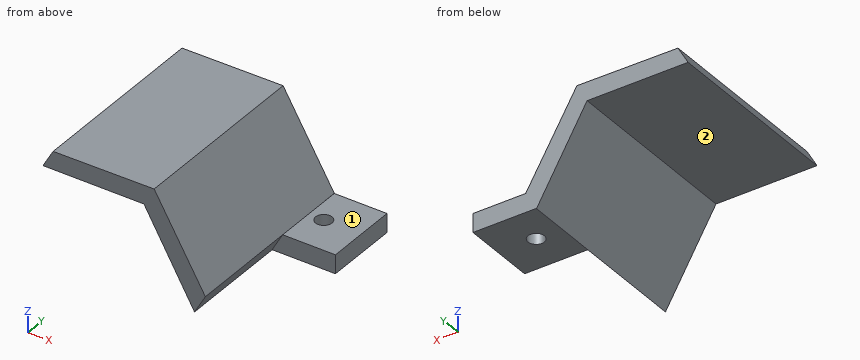
```python
from build123d import *

# Parameters (mm, degrees)
ESQUISSE3_W             = 20
ESQUISSE3_H             = 20
BOSS_EXTRU_2_DEPTH      = 5
ESQUISSE5_R             = 2.2
ENL_V_MAT_EXTRU_2_DEPTH = 5
BOSS_EXTRU_4_DEPTH      = 1
BOSS_EXTRU_4_DEPTH_BACK = 50
ENL_V_MAT_EXTRU_3_DEPTH = 52
ESQUISSE17_W            = 44.772761967
ESQUISSE17_H            = 32.67201549
ENL_V_MAT_EXTRU_4_DEPTH = 1


with BuildPart() as part:
    # Esquisse3 → Boss.-Extru.2 (new body)
    with BuildSketch(Plane.XY):
        with Locations((0.833384448, -1.552723646)):
            Rectangle(ESQUISSE3_W, ESQUISSE3_H)
    extrude(amount=BOSS_EXTRU_2_DEPTH)

    # Esquisse5 → Enlèv. mat.-Extru.2 (cut)
    with BuildSketch(Plane.XY.offset(5)):
        with Locations((0.833384448, -1.552723646)):
            Circle(ESQUISSE5_R)
    extrude(amount=-ENL_V_MAT_EXTRU_2_DEPTH, mode=Mode.SUBTRACT)

    # Esquisse15 → Boss.-Extru.4 (add, two sides: drawn at the far end of the back side and taken through both)
    with BuildSketch(Plane(origin=(0, 8.447276354, 0), x_dir=(1, 0, 0), z_dir=(0, 1, 0)).offset(-BOSS_EXTRU_4_DEPTH_BACK)):
        Polygon((-16.923746628, -28.293399859), (-3.242841841, -5.019846719), (-16.557877703, 18.464940943), (-43.553818352, 18.676175465), (-57.234723139, -4.597377675), (-43.919687277, -28.082165337), align=None)
    extrude(amount=BOSS_EXTRU_4_DEPTH + BOSS_EXTRU_4_DEPTH_BACK)

    # Esquisse16 → Enlèv. mat.-Extru.3 (cut)
    with BuildSketch(Plane(origin=(0, 9.447276354, 0), x_dir=(1, 0, 0), z_dir=(0, 1, 0))):
        Polygon((-3.971698256, 3.828685124), (-19.643043748, 30.972251739), (-50.985734731, 30.972251739), (-66.657080223, 3.828685124), (-50.985734731, -23.314881491), (-19.643043748, -23.314881491), align=None)
    extrude(amount=-ENL_V_MAT_EXTRU_3_DEPTH, mode=Mode.SUBTRACT)

    # Esquisse17 → Enlèv. mat.-Extru.4 (cut)
    with BuildSketch(Plane(origin=(0, 9.447276354, 0), x_dir=(1, 0, 0), z_dir=(0, 1, 0))):
        with Locations((-25.155039142, -14.317707157)):
            Rectangle(ESQUISSE17_W, ESQUISSE17_H)
    extrude(amount=-ENL_V_MAT_EXTRU_4_DEPTH, mode=Mode.SUBTRACT)


solid = part.part
```
Input: part model. Units: mm. Frame: model coordinates. Face numbers are marked on the shaded views. A direction names the side the tool comes from. Coordinates: 2 decimals unless noted, no trailing zeros. Order: outer loops, then holes, each group sorted by start corner. A loop starts at its lowest first (then second) coordinate and runs counter-clockwise, first axis right, second up. Notation, with made-up numbers: (29.5, 71.25) - (41.5, 71.25) arc R23 cw to (41.5, 80.25) - close; hole circle Ø6 at (23.25, 56). An arc over 180 degrees is marked (long way). Put each result on its own line as item: value.
1. Cut plane B-B on x = -4.5. Return the cut outline in (y, z), then the cut area to 3 significant figures.
Report:
outline: (-41.55, 2.8) - (-11.55, 2.8) - (-11.55, 0) - (8.45, 0) - (8.45, 7.16) - (-41.55, 7.16) - close
area: 274 mm2
2. Line query: line 1 along Z through (x, y) = (-42, -12.5); line 2 along Y through (x, z) = (8, 3); line 3 along Z through (x, y) = (-16.5, -15). Output: solid intervals per line, ascending.
Report:
line 1: z = 23.31 to 28.1
line 2: y = -11.55 to 8.45
line 3: z = 17.87 to 27.57
3. Cut plane A-A on y = -32. Return the cut outline in (x, z), then the cut area to 3 significant figures.
Report:
outline: (-46.62, 23.31) - (-19.64, 23.31) - (-6.14, -0.08) - (-3.24, 5.02) - (-16.92, 28.29) - (-43.92, 28.08) - close
area: 265 mm2
4. Reachability of the marked faces 1 and 2 from +Z, -Z, +X, -X, +Y, -Y: full face, straight path, thin tool, end or side. Return the list, or none.
Report:
face 1: +Z, +X, +Y, -Y
face 2: -Z, -X, +Y, -Y
5. Contact query for flat-ended pins moving along their axis: pin 1 Ø12 at (x, y) = (-36.5, -14.5) entering from +Z; pin 2 Ø1 at (x, z) = (-7.5, 13) entering from -Y; pin 3 Ø2.5 at (x, z) = (-1, 2.5) entering from -Y; pin 4 Ø2 at (y, z) = (-10, 20.5) entering from +X. Output: stop coordinate, or through.
Report:
pin 1: stops at z = 28.19
pin 2: stops at y = -41.55
pin 3: stops at y = -11.55
pin 4: stops at x = -11.75
6. Cut plane D-D on z = 7. Return the cut outline in (x, y).
Report:
outline: (-10.22, -41.55) - (-4.41, -41.55) - (-4.41, 8.45) - (-10.22, 8.45) - close
